Autodesk Inventor part; units mm, degrees
ref_plane "YZ Plane" through (0, 0, 0) normal (1, 0, 0) x (0, 1, 0)
ref_plane "XZ Plane" through (0, 0, 0) normal (0, 1, 0) x (-1, 0, 0)
ref_plane "XY Plane" through (0, 0, 0) normal (0, 0, 1) x (1, 0, 0)
sketch "スケッチ1" plane through (0, 0, 0) normal (0, 1, 0) x (-1, 0, 0)
  circle A0 centre (0, 0) radius 12
  line L0 (18, 10) -> (-18, 10)
  line L1 (-18, 10) -> (-18, -18)
  line L2 (-18, -18) -> (18, -18)
  line L3 (18, -18) -> (18, 10)
  line L4 (18, 30) -> (-18, 30)
  line L5 (-18, 30) -> (-18, 10)
  line L6 (-18, 10) -> (18, 10)
  line L7 (18, 10) -> (18, 30)
  line L8 (18, 30) -> (-18, 10) construction
  line L9 (-18, 30) -> (18, 10) construction
  point P0 (0, 20)
  point P1 (0, 20)
  point P2 (20, 10)
  point P3 (-6.6332, 10)
  point P4 (6.6332, 10)
  dimension "d0" = 24
  dimension "d18" = 10
  dimension "d33" = 30
  dimension "d34" = 36
  dimension "d36" = 18
extrude "押し出し1" add sketch "スケッチ1" along normal mid plane 10 contours A0 L0 L3 L2 L1 | A0 L0 L5 L4 L7
sketch "スケッチ2" plane through (-38, 5, 30) normal (0, 0, 1) x (1, 0, 0)
  line L0 (20, -10) -> (20, 0)
  line L1 (56, -10) -> (20, -10)
  line L2 (56, 0) -> (56, -10)
  point P0 (38, -5)
  point P1 (25, -5)
  point P2 (51, -5)
  dimension "d37" = 5
  dimension "d38" = 5
  dimension "d39" = 5
hole "穴1" at (-13, 0, 30) at (13, 0, 30) direction (0, 0, -1) diameter 5 depth 6 tip angle 118
fillet "フィレット1" radius 10 4 edges at (18, 2.5, -18) (18, -2.5, -18) (-18, 2.5, -18) (-18, -2.5, -18)
chamfer "面取り1" distance 1 angle 45 2 edges at (5.6745, 5, -10.5735) (0, 5, 12)
properties part number "cable_holder" material "ABS プラスチック"
Build history of the part. All positions in model axes, mm. A direction names the side the tool comes from. Round coordinates to 2 decimals unless told otherwise and drop trailing zeros. Write each loop counter-clockwise with the first axis right and the second up, starting at its lowest first coordinate (ties: lowest second). Pieces come first, ordered by that corner, then holes. Notation, with made-up numbers: M -13,44 L 25,44 A30 ccw 25,74 Z; hole C -5.5,9.25 d11. An arc over 180 degrees is marked long. Answer as a JSON object with one key per item and string values. Group by question number.
(1) Flat gauge pins, fed straight in: pin 1 (10 mm diameter, centred on x = 3, z = 6, fed in from -Y); pin 2 (4 mm diameter, centred on y = -1.5, z = -12, fed in from -X); pin 3 (4.5 mm diameter, centred on x = 13, y = 0, fed in from +Z). Where does each tip first touch, or does it go through?
(2) Drill centre lines: L1, parallel to X at y = 0, z = 25.8; L2, parallel to Y at x = 13, z = 26; L3, parallel to Z at x = -10, y = 2.75. Where is each one in solid material? Low to high.
(3) Which spindle directions (+Z, -Z, +X, -X, +Y, -Y) get a long thin tool onto all of the face, cutting with end or side? Do faces 1 (the cylindrical face through (-10.56, 0.54, 26.96)), 2 (the flat face through (4, -5, 12)). Say none if no direction does.
(4) Cut at B-B (x = 0). Give the cut face in (y, z).
(5) Mould opens along Y. For faces 3 (the flat face through (18, 0, 11)), 4 (the flat face through (0, 5, 17)), 5 (the cylindrical face through (15.44, 0.54, 26.96)), 6 (the conical face through (13.37, -0.23, 22.76)) say: pulls with the +Y half, pulls with the -Y half, needs draft (parallel to the pull), parting line crosses it, or undercut.
(6) Cut at A-A (z = 0). Give the cut face in (x, y), and give its area (3 significant figures).
Responses:
{
 "1": {"pin 1": "passes through", "pin 2": "stops at x = -17.8", "pin 3": "stops at z = 23.85"},
 "2": {"L1": "x = -18 to -15.5, -10.5 to 10.5, 15.5 to 18", "L2": "y = -5 to -2.5, 2.5 to 5", "L3": "z = -17.8 to -6.63, 6.63 to 30"},
 "3": {"face 1": "+Z", "face 2": "+Z, -Z, +X, -X, -Y"},
 "4": {"outline": "M -5,-18 L 5,-18 L 5,-13 L 4,-12 L -5,-12 Z; M -5,12 L 4,12 L 5,13 L 5,30 L -5,30 Z"},
 "5": {"face 3": "needs draft", "face 4": "pulls with the +Y half", "face 5": "undercut", "face 6": "undercut"},
 "6": {"outline": "M -18,-5 L -12,-5 L -12,4 L -13,5 L -18,5 Z; M 12,-5 L 18,-5 L 18,5 L 13,5 L 12,4 Z", "area": "119 mm2"}
}
